from build123d import *

# Parameters (mm, degrees)
BOSS_EXTRUDE1_DEPTH = 20
SKETCH2_W           = 10
SKETCH2_H           = 50
BOSS_EXTRUDE2_DEPTH = 100
SKETCH4_R           = 4
CUT_EXTRUDE2_DEPTH  = 125.599357944
FILLET1_R           = 5
SKETCH7_R           = 4
CUT_EXTRUDE3_DEPTH  = 142.155942135
BOSS_EXTRUDE3_DEPTH = 50
FILLET2_R           = 10
BOSS_EXTRUDE4_DEPTH = 50
FILLET3_R           = 10


with BuildPart() as part:
    # Sketch1 → Boss-Extrude1 (new body)
    with BuildSketch(Plane(origin=(0, 0, 0), x_dir=(1, 0, 0), z_dir=(0, 1, 0))):
        Polygon((-25, 45), (-25, 30), (-25, -30), (-25, -50), (15, -50), (15, -30), (15, 30), (15, 70), (-25, 70), align=None)
    extrude(amount=BOSS_EXTRUDE1_DEPTH)

    # Sketch2 → Boss-Extrude2 (add)
    with BuildSketch(Plane(origin=(0, 20, 0), x_dir=(1, 0, 0), z_dir=(0, 1, 0))):
        with Locations((-5, 10)):
            Rectangle(SKETCH2_W, SKETCH2_H)
    extrude(amount=BOSS_EXTRUDE2_DEPTH)

    # Sketch4 → Cut-Extrude2 (cut, through all)
    with BuildSketch(Plane(origin=(0, 20, 0), x_dir=(1, 0, 0), z_dir=(0, 1, 0))):
        with Locations(Location((-5, 55, 0), (0, 0, 270))):
            Circle(SKETCH4_R)
        with Locations(Location((-5, -35, 0), (0, 0, 270))):
            Circle(SKETCH4_R)
    extrude(amount=-CUT_EXTRUDE2_DEPTH, mode=Mode.SUBTRACT)

    # Fillet1
    fillet1_edges = [part.edges().sort_by_distance(p)[0] for p in [
        (-25, 10, -70),
        (15, 10, -70),
        (15, 10, 50),
        (-25, 10, 50),
        (-5, 120, 15),
        (-5, 120, -35),
    ]]
    fillet(fillet1_edges, radius=FILLET1_R)

    # Sketch7 → Cut-Extrude3 (cut, through all)
    with BuildSketch(Plane.ZY.offset(10)):
        with Locations((-25, 110)):
            Circle(SKETCH7_R)
        with Locations((5, 110)):
            Circle(SKETCH7_R)
    extrude(amount=-CUT_EXTRUDE3_DEPTH, mode=Mode.SUBTRACT)

    # Sketch9 → Boss-Extrude3 (add)
    with BuildSketch(Plane.XY.offset(15)):
        Polygon((-10, 20), (-25, 20), (-10, 70), align=None)
    extrude(amount=-BOSS_EXTRUDE3_DEPTH)

    # Fillet2
    fillet2_edges = [part.edges().sort_by_distance(p)[0] for p in [
        (-10, 70, -10),
    ]]
    fillet(fillet2_edges, radius=FILLET2_R)

    # Sketch10 → Boss-Extrude4 (add)
    with BuildSketch(Plane.XY.offset(15)):
        Polygon((0, 20), (15, 20), (0, 70), align=None)
    extrude(amount=-BOSS_EXTRUDE4_DEPTH)

    # Fillet3
    fillet3_edges = [part.edges().sort_by_distance(p)[0] for p in [
        (0, 70, -10),
    ]]
    fillet(fillet3_edges, radius=FILLET3_R)


solid = part.part
The listing builds one solid part. Answer for the finished solid, in the listing's coordinates (mm). A direction names the side the tool comes from. Coordinates: 2 decimals unless noted, no trailing zeros. Write each loop counter-clockwise with the first axis right and the second up, starting at its lowest first coordinate (ties: lowest second). Pieces come first, ordered by that corner, then holes. Notation, with made-up numbers: (-11, 87) - (25, 87) arc R23 cw to (25, 121) - close; hole circle Ø1 at (14, 88). An arc over 180 degrees is marked (long way). Answer as CSV lines item,"result".
1. Find section A-A (z = -55). Give the vertices of the cut face in (x, y).
Computed values:
outline,"(-25, 0) - (-9, 0) - (-9, 20) - (-25, 20) - close; (-1, 0) - (15, 0) - (15, 20) - (-1, 20) - close"
2. Find section D-D (z = -25). Give the vertices of the cut face in (x, y).
Computed values:
outline,"(-25, 0) - (15, 0) - (15, 20) - (0.42, 68.59) arc R10 cw to (0, 71.47) - (0, 106) - (-10, 106) - (-10, 71.47) arc R10 cw to (-10.42, 68.59) - (-25, 20) - close; (-10, 114) - (0, 114) - (0, 120) - (-10, 120) - close"
3. A tool of negligible diameter and unlimited length cuts with its end or side. For faces 4 (the flat face through (-17.8, 44, -9.6)), 5 (the flat face through (-5, 58, 15)), 6 (the flat face through (-5, 20, -49)), from which of +Z, -Z, +X, -X, +Y, -Y can it reach the whole face along a straight path? Write none if from no direction.
Computed values:
face 4,"+Z, -Z, -X, +Y"
face 5,"+Z, +X, -X, +Y"
face 6,"-Z, +X, -X, +Y"
4. Straight lines are drawn through the part: line 1 (Y direction, x = -7, z = -63.5); line 2 (Z direction, x = -8, y = 29); line 3 (Y direction, x = -7, z = 5). For each, find the intervals that lie inside material, in ascending order. Write a range as [from, to].
Computed values:
line 1,"y = [0, 20]"
line 2,"z = [-35, 15]"
line 3,"y = [0, 106], [114, 120]"
5. Determine the mould class of faces 1 (the cylindrical face through (-5.07, 113.966, 4.479)), 2 (the cylindrical face through (-5, 118, -34)), 3 (the cylindrical face through (-23, 10, 49)) for opening direction Y: +Y half, -Y half, draft (parallel to the pull), parting line (faces both ways), or undercut.
Computed values:
face 1,"undercut"
face 2,"+Y half"
face 3,"draft"
6. Find section B-B (x = -5). Give the vertices of the cut face in (y, z), plus the area to 3 significant figures.
Computed values:
outline,"(0, -70) - (20, -70) - (20, -59) - (0, -59) - close; (0, -51) - (20, -51) - (20, -35) - (115, -35) arc R5 ccw to (120, -30) - (120, 10) arc R5 ccw to (115, 15) - (20, 15) - (20, 31) - (0, 31) - close; (0, 39) - (20, 39) - (20, 50) - (0, 50) - close; hole circle Ø8 at (110, -25); hole circle Ø8 at (110, 5)"
area,"6,970 mm²"
7. Given P1, Ø14.5, axis at y = 90, z = -18, coming from the -X side; P2, Ø12, axis at x = -13.5, y = 70.5, coming from the -Z side; P3, Ø12, axis at x = 3.5, y = 66.5, coming from the +Z side; P4, Ø6.5, axis at x = -5, z = -55, coming from the -Y side, each flat-ended and moving along its own axis, determine where each tip first touches the part or whether it passes through.
Computed values:
P1,"stops at x = -10"
P2,"stops at z = -35"
P3,"stops at z = 15"
P4,"passes through"
8. Find section C-C (y = 12.5). Give the vertices of the cut face in (x, z), plus the area to 3 significant figures.
Computed values:
outline,"(-25, -65) arc R5 ccw to (-20, -70) - (10, -70) arc R5 ccw to (15, -65) - (15, 45) arc R5 ccw to (10, 50) - (-20, 50) arc R5 ccw to (-25, 45) - close; hole circle Ø8 at (-5, -55); hole circle Ø8 at (-5, 35)"
area,"4,680 mm²"
